Source: CAD feature listing. Evaluate the final solid. Frame: model axes, mm. A direction names the side the tool comes from. Round coordinates to 2 decimals unless told otherwise and drop trailing zeros. Loops run counter-clockwise (first coordinate to the right, second up) from the corner with the lowest first, then second, coordinate; pieces in that order, holes last. Notation, with made-up numbers: M 72,-3.75 L 79,-3.75 A37 ccw 79,32.25 Z; hole C 31.5,84.25 d3. An arc over 180 degrees is marked long. Answer as a JSON object with one key per item and string values.
from build123d import *

# Parameters (mm, degrees)
SKETCH1_R           = 1.8288
BOSS_EXTRUDE1_DEPTH = 3.302
SKETCH2_R           = 1.5
CUT_EXTRUDE1_DEPTH  = 4.302
SKETCH3_R           = 1.524
SKETCH3_W           = 10.16
SKETCH3_H           = 3.175
CUT_EXTRUDE2_DEPTH  = 4.302


with BuildPart() as part:
    # Sketch1 → Boss-Extrude1 (new body)
    with BuildSketch(Plane(origin=(0, 0, 0), x_dir=(1, 0, 0), z_dir=(0, 1, 0))):
        Polygon((-164.846, 76.2), (-139.446, 76.2), (-139.446, 63.5), (-133.096, 63.5), (-133.096, 76.2), (-31.75, 76.2), (-31.75, 63.5), (-25.4, 63.5), (-25.4, 76.2), (0, 76.2), (0, 48.895), (-3.175, 48.895), (-3.175, 27.305), (0, 27.305), (0, 0), (-25.4, 0), (-25.4, 12.7), (-31.75, 12.7), (-31.75, 0), (-133.096, 0), (-133.096, 12.7), (-139.446, 12.7), (-139.446, 0), (-164.846, 0), (-164.846, 27.305), (-164.846, 48.895), align=None)
        with Locations((-82.423, 38.1)):
            Circle(SKETCH1_R, mode=Mode.SUBTRACT)
    extrude(amount=BOSS_EXTRUDE1_DEPTH)

    # Sketch2 → Cut-Extrude1 (cut, through all)
    with BuildSketch(Plane(origin=(0, 3.302, 0), x_dir=(1, 0, 0), z_dir=(0, 1, 0))):
        with Locations((-158.496, 30.35)):
            Circle(SKETCH2_R)
        with Locations((-158.496, 6.35)):
            Circle(SKETCH2_R)
        with Locations((-64.496, 6.35)):
            Circle(SKETCH2_R)
        with Locations((-64.496, 30.35)):
            Circle(SKETCH2_R)
    extrude(amount=-CUT_EXTRUDE1_DEPTH, mode=Mode.SUBTRACT)

    # Sketch3 → Cut-Extrude2 (cut, through all)
    with BuildSketch(Plane(origin=(0, 3.302, 0), x_dir=(1, 0, 0), z_dir=(0, 1, 0))):
        with Locations((-73.406, 51.723686304)):
            Circle(SKETCH3_R)
        with Locations((-122.169322677, 38.81724188)):
            Rectangle(SKETCH3_W, SKETCH3_H)
        with Locations((-122.169322677, 72.47224188)):
            Rectangle(SKETCH3_W, SKETCH3_H)
    extrude(amount=-CUT_EXTRUDE2_DEPTH, mode=Mode.SUBTRACT)


solid = part.part
Item 1: Section D-D on y = 2. Give the number of separate pieces and of enclosed holes in the cut face, then the cut area to 3 significant figures.
Answer sheet:
{"separate pieces": "1", "enclosed holes": "8", "area": "12,100 mm²"}
Item 2: Access query for faces 5 (the flat face through (-139.446, 2, -6)), 6 (the flat face through (-139.446, 2, -70)), 7 (the flat face through (-2, 2, -27.305)), 8 (the flat face through (-127.249, 2, -72)). Directions: +Z, -Z, +X, -X, +Y, -Y. A direction counts if a zero-diameter tool reaches every point of the face in a straight line with its end or side. Return the directions, or none.
Answer sheet:
{"face 5": "+Z, +Y, -Y", "face 6": "-Z, +Y, -Y", "face 7": "+X, +Y, -Y", "face 8": "+Y, -Y"}
Item 3: Pull-direction query (Z, two-part tool) for faces 1 (the cylindrical face through (-157.1, 1.7, -5.8)), 2 (the cylindrical face through (-63.065, 1.674, -6.801)), 3 (the flat face through (-31.75, 2, -6)), 4 (the flat face through (-29, 2, -12.7)); classes: pulls with the +Z half, pulls with the -Z half, needs draft (parallel to the pull), parting line crosses it, or undercut.
Answer sheet:
{"face 1": "undercut", "face 2": "undercut", "face 3": "needs draft", "face 4": "pulls with the +Z half"}
Item 4: Section B-B on z = -6.35. Return the cut outline in (x, y).
Answer sheet:
{"outline": "M -164.85,0 L -160,0 L -160,3.3 L -164.85,3.3 Z; M -157,0 L -139.45,0 L -139.45,3.3 L -157,3.3 Z; M -133.1,0 L -66,0 L -66,3.3 L -133.1,3.3 Z; M -63,0 L -31.75,0 L -31.75,3.3 L -63,3.3 Z; M -25.4,0 L 0,0 L 0,3.3 L -25.4,3.3 Z"}
Item 5: Line query: probe 1 along X at (y, z) = (1.1, -6.35); probe 2 along X at (y, z) = (0.5, -70); probe 3 along X at (y, z) = (1.9, -30.35) (3 decimals). Output: solid intervals per line, ascending. Write a range as from..to.
Answer sheet:
{"probe 1": "x = -164.85..-160, -157..-139.45, -133.1..-66, -63..-31.75, -25.4..0", "probe 2": "x = -164.85..-139.45, -133.1..-31.75, -25.4..0", "probe 3": "x = -164.846..-159.996, -156.996..-65.996, -62.996..-3.175"}
Item 6: Section A-A on x = -123.5. Return the cut outline in (y, z), then the cut area to 3 significant figures.
Answer sheet:
{"outline": "M 0,-76.2 L 3.3,-76.2 L 3.3,-74.06 L 0,-74.06 Z; M 0,-70.88 L 3.3,-70.88 L 3.3,-40.4 L 0,-40.4 Z; M 0,-37.23 L 3.3,-37.23 L 3.3,0 L 0,0 Z", "area": "231 mm²"}
Item 7: Section C-C on z = -30.35. Return the cut outline in (x, y) (3 decimals).
Answer sheet:
{"outline": "M -164.846,0 L -159.996,0 L -159.996,3.302 L -164.846,3.302 Z; M -156.996,0 L -65.996,0 L -65.996,3.302 L -156.996,3.302 Z; M -62.996,0 L -3.175,0 L -3.175,3.302 L -62.996,3.302 Z"}
Item 8: Contact query for a flat-ended pin moving along its axis: pin 1 Ø6 at (x, z) = (-53, -33) entering from -Y. Output: stop coordinate, or through.
Answer sheet:
{"pin 1": "stops at y = 0"}
